from build123d import *

# Parameters (mm, degrees)
F0_R     = 10.9
F1_DEPTH = 25


with BuildPart() as f1:
    # F0 (on Front) → F1 (new body)
    with BuildSketch(Plane.XZ):
        with BuildLine():
            Line((-4.909692, 34.903756), (-8.6357, 8.698229))
            ThreePointArc((-8.6357, 8.698229), (-10.61489, 6.128509), (-11.850737, 3.129621))
            Line((-11.850737, 3.129621), (-32.682386, -13.19996))
            Line((-32.682386, -13.19996), (-30.22754, -17.451878))
            Line((-30.22754, -17.451878), (-27.772694, -21.703796))
            Line((-27.772694, -21.703796), (-3.215038, -11.82785))
            ThreePointArc((-3.215038, -11.82785), (0, -12.257019), (3.215038, -11.82785))
            Line((3.215038, -11.82785), (27.772694, -21.703796))
            Line((27.772694, -21.703796), (30.22754, -17.451878))
            Line((30.22754, -17.451878), (32.682386, -13.19996))
            Line((32.682386, -13.19996), (11.850737, 3.129621))
            ThreePointArc((11.850737, 3.129621), (10.61489, 6.128509), (8.6357, 8.698229))
            Line((8.6357, 8.698229), (4.909692, 34.903756))
            Line((4.909692, 34.903756), (0, 34.903756))
            Line((0, 34.903756), (-4.909692, 34.903756))
        make_face()
        Polygon((-16.33297, -15.897677), (-21.934277, -13.029107), (-22.250676, -6.743948), (-16.965768, -3.327359), (-11.364461, -6.195929), (-11.048062, -12.481088), align=None, mode=Mode.SUBTRACT)
        Polygon((21.934277, -6.195929), (22.250676, -12.481088), (16.965768, -15.897677), (11.364461, -13.029107), (11.048062, -6.743948), (16.33297, -3.327359), align=None, mode=Mode.SUBTRACT)
        Circle(F0_R, mode=Mode.SUBTRACT)
        Polygon((5.601307, 16.356466), (0.316399, 12.939876), (-5.284908, 15.808446), (-5.601307, 22.093605), (-0.316399, 25.510195), (5.284908, 22.641625), align=None, mode=Mode.SUBTRACT)
    extrude(amount=F1_DEPTH)


solid = f1.part
The listing builds one solid part. Answer for the finished solid, in the listing's coordinates (mm). A direction names the side the tool comes from. Give positions to 0.01 mm unless a question says otherwise; leave off trailing zeros. Write each loop counter-clockwise with the first axis right and the second up, starting at its lowest first coordinate (ties: lowest second). Pieces come first, ordered by that corner, then holes. Notation, with made-up numbers: (-6.75, 58.5) - (44.25, 58.5) arc R17 ccw to (44.25, 90.5) - close; hole circle Ø6 at (-6, -28). An arc over 180 degrees is marked (long way). Use a Markdown table: item, result.
1. A tool of negligible diameter and unlimited length cuts with its end or side. For faces 4 (the flat face through (-19.645, -12.325, -5.06)), 5 (the flat face through (-6.747, -12.325, 21.984)), from which of +Z, -Z, +X, -X, +Y, -Y can it reach the whole face along a straight path? Write none if from no direction.
Values follow:
| item | result |
|---|---|
| face 4 | +Y, -Y |
| face 5 | +Z, -X, +Y, -Y |
2. Each of these flat-tipped pins is pushed along its axis until it touches: P1, Ø2, axis at y = -16.5, z = 22, coming from the -X side; P2, Ø12, axis at x = -11, z = 27, coming from the +Y side; P3, Ø6, axis at x = 18.5, y = -16.5, coming from the +Z side; P4, Ø1.5, axis at y = -16, z = 27, coming from the -X side. Where does it stop, or does it pass through?
Values follow:
| item | result |
|---|---|
| P1 | stops at x = -6.89 |
| P2 | stops at y = 0 |
| P3 | stops at z = 0.27 |
| P4 | stops at x = -6.14 |
3. For a pull along Z with two mould halves and no side action, classify faces 1 (the flat face through (13.65, -12.32, -5.06)), 2 (the cylindrical face through (10.638, -12.325, 6.089)), 3 (the flat face through (-15.666, -12.325, -16.835)) as released by +Z, released by -Z, zero draft, split by the parting line, or undercut.
Values follow:
| item | result |
|---|---|
| face 1 | undercut |
| face 2 | released by +Z |
| face 3 | released by -Z |
4. Section B-B on z = 0 is taken. Write down the section's boundary in (x, y), plus the area to 3 significant figures.
Values follow:
| item | result |
|---|---|
| outline | (-15.84, -25) - (-10.9, -25) - (-10.9, 0) - (-15.84, 0) - close; (10.9, -25) - (15.84, -25) - (15.84, 0) - (10.9, 0) - close |
| area | 247 mm² |
5. Section D-D on x = 21 is taken. Write down the section's boundary in (y, z).
Values follow:
| item | result |
|---|---|
| outline | (-25, -18.98) - (0, -18.98) - (0, -13.29) - (-25, -13.29) - close; (-25, -5.72) - (0, -5.72) - (0, -4.04) - (-25, -4.04) - close |
6. Section C-C on y = -7.5 is taken. Count the separate pieces of the cut face and the enclosed holes in it, plus the area to 3 significant figures.
Values follow:
| item | result |
|---|---|
| separate pieces | 1 |
| enclosed holes | 4 |
| area | 728 mm² |
7. Find the intervals of material crossed by probe 1 along Z at (x, y) = (0, -13.25); probe 2 along X at (y, z) = (-11.75, -6.5); probe 3 along Z at (x, y) = (-4.5, -11.5), in increasing order. Write a range as from..to.
Values follow:
| item | result |
|---|---|
| probe 1 | z = -12.26..-10.9, 10.9..13.1, 25.35..34.9 |
| probe 2 | x = -24.14..-21.87, -11.35..-8.75, 8.75..11.43, 21.95..24.14 |
| probe 3 | z = -12.34..-9.93, 9.93..15.41, 22.81..34.9 |
8. Section A-A on x = -4 is taken. Write down the section's boundary in (y, z), plus the area to 3 significant figures.
Values follow:
| item | result |
|---|---|
| outline | (-25, -12.14) - (0, -12.14) - (0, -10.14) - (-25, -10.14) - close; (-25, 10.14) - (0, 10.14) - (0, 15.15) - (-25, 15.15) - close; (-25, 23.13) - (0, 23.13) - (0, 34.9) - (-25, 34.9) - close |
| area | 470 mm² |
